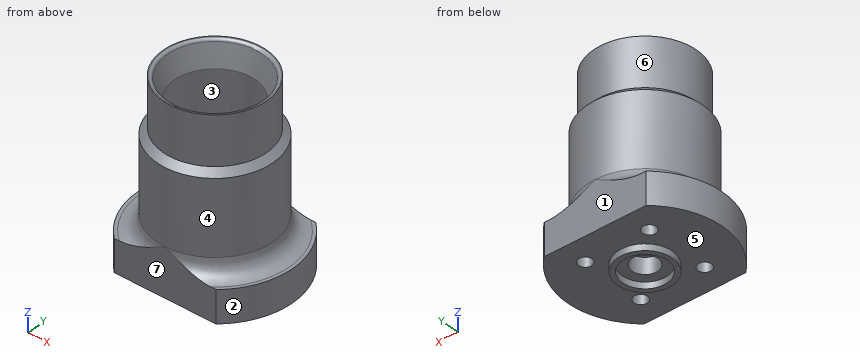
```python
from build123d import *

# Parameters (mm, degrees)
F2_W     = 70
F2_H     = 56
F2_W_2   = 65
F2_H_2   = 36
F3_DEPTH = 57.001
F5_D     = 4.2
F5_DEPTH = 14
F5_TIP   = 1.2618073


with BuildPart() as f1:
    # F0 (on Front) → F1 (revolve)
    with BuildSketch(Plane.XZ):
        with BuildLine():
            Line((4, 7), (4, 2))
            Line((4, 2), (7, 2))
            Line((7, 2), (7, 0))
            Line((7, 0), (8.5, 0))
            Line((8.5, 0), (8.5, 2))
            Line((8.5, 2), (24, 2))
            Line((24, 2), (24, 12))
            Line((24, 12), (23, 12))
            ThreePointArc((23, 12), (19.4644660941, 13.4644660941), (18, 17))
            Line((18, 17), (18, 40))
            Line((18, 40), (16, 42))
            Line((16, 42), (16, 57))
            Line((16, 57), (15.7047191962, 57))
            ThreePointArc((15.7047191962, 57), (15.1286707595, 56.8174155605), (14.7629772846, 56.336336397))
            Line((14.7629772846, 56.336336397), (12.5, 50))
            Line((12.5, 50), (12.5, 23))
            Line((12.5, 23), (2.25, 23))
            Line((2.25, 23), (2.25, 7))
            Line((2.25, 7), (4, 7))
        make_face()
    revolve(axis=Axis((0, 0, 40.597807616), (0, 0, 1)))

    # F2 (on Top) → F3 (cut, through all)
    with BuildSketch(Plane.XY):
        Rectangle(F2_W, F2_H)
        Rectangle(F2_W_2, F2_H_2, mode=Mode.SUBTRACT)
    extrude(amount=F3_DEPTH, mode=Mode.SUBTRACT)

    # F5
    with Locations(Plane(origin=(0, 0, 2), x_dir=(1, 0, 0), z_dir=(0, 0, -1))):
        with Locations((-9.998489886, 9.998489886), (9.998489886, 9.998489886), (9.998489886, -9.998489886), (-9.998489886, -9.998489886)):
            Hole(F5_D / 2, depth=F5_DEPTH)
            with Locations((0, 0, -(F5_DEPTH + F5_TIP / 2))):  # 118° drill point
                Cone(0, F5_D / 2, F5_TIP, mode=Mode.SUBTRACT)


solid = f1.part
```
Model file for the job. Use its own axes, mm. Face numbers are marked on the shaded views. A direction names the side the tool comes from. Coordinates: 2 decimals unless noted, no trailing zeros. Loops run counter-clockwise (first coordinate to the right, second up) from the corner with the lowest first, then second, coordinate; pieces in that order, holes last. Notation, with made-up numbers: (29.5, 5) - (66.5, 5) arc R17 ccw to (66.5, 15) - close; hole circle Ø10 at (-20.5, 30.5). An arc over 180 degrees is marked (long way). Write item = value, one per line. Start each with the question number.
Item 1: Wall check: probe 1 along Z at (x, y) = (-9.5, 7); probe 2 along Y at (x, z) = (5.5, 42); probe 3 along Y at (x, z) = (10.5, 27). Give the ranges that are in metal, low to high. Write a range as [from, to].
Item 2: Drop flat-ended pins along their axis: pin 1 Ø10 at (x, z) = (-17, 51) entering from +Y; pin 2 Ø12 at (y, z) = (11.5, 9.5) entering from -X; pin 3 Ø5 at (x, z) = (-16, 28) entering from -Y; pin 4 Ø2.5 at (x, y) = (0, 0) entering from -Z. Give the stop position or say it passes through.
Item 3: Saw through at B-B, the plane z = 32. List the corners of the cut face in (x, y), then the cut area to 3 significant figures.
Item 4: 3-axis set-ups, long thin cutter, end or side, ignore diameter. For the marked faces 5, 6 and 7: which of +Z, -Z, +X, -X, +Y, -Y reach the whole face in a straight line?
Item 5: Saw through at A-A, the plane z = 44. List the corners of the cut face in (x, y), then the cut area to 3 significant figures.
Item 6: Pull direction X, two halves, no side cores. Call the marked faces 1, 2, 3 and 4: +X half, -X half, draft (parallel to the pull), parting line (faces both ways), or undercut.
Answers:
q1.probe_1 = [2, 23]
q1.probe_2 = [-15.02, -11.22], [11.22, 15.02]
q1.probe_3 = [-14.62, -6.78], [6.78, 14.62]
q2.pin_1 = 10.58
q2.pin_2 = -23.36
q2.pin_3 = -11.91
q2.pin_4 = through
q3.outline = circle Ø36 at (0, 0); hole circle Ø25 at (0, 0)
q3.area = 527 mm2
q4.face_5 = -Z
q4.face_6 = +Z
q4.face_7 = +Z, -Z, +X, -X, -Y
q5.outline = circle Ø32 at (0, 0); hole circle Ø25 at (0, 0)
q5.area = 313 mm2
q6.face_1 = draft
q6.face_2 = +X half
q6.face_3 = undercut
q6.face_4 = parting line
